The model under review builds one solid part; all positions refer to its coordinate system, in mm. A direction names the side the tool comes from. Round coordinates to 2 decimals unless told otherwise and drop trailing zeros. Write each loop counter-clockwise with the first axis right and the second up, starting at its lowest first coordinate (ties: lowest second). Pieces come first, ordered by that corner, then holes. Notation, with made-up numbers: M 4,54 L 10,54 A26 ccw 10,68 Z; hole C -18,38 d8. An arc over 180 degrees is marked long. Write item = value, one per line. Start each with the question number.
Item 1: Take a section at B-B, the plane y = 3.5. Give the boundary of the cut face in (x, z).
Item 2: Tool access review of faces 4 (the flat face through (0, 5, 0)), 5 (the flat face through (-1, 15, -14)), 6 (the cylindrical face through (17.553, 10.267, -2.764)): name each direction out of +Z, -Z, +X, -X, +Y, -Y from which nothing blocks a thin tool from reaching the whole face with its end or side.
Item 3: To check wall thickness, follow line 1 along X through (y, z) = (2.6, 0); line 2 along X through (y, z) = (7, 11.5); line 3 along X through (y, z) = (5.75, -7.5). State the ranges of each line that lie inside material, in increasing order.
Item 4: For pin 1 Ø5 at (x, z) = (38.5, -11.5) entering from -Y; pin 2 Ø3 at (x, z) = (61.5, 1) entering from -Y; pin 3 Ø13 at (x, z) = (60, 0) entering from +Y; pin 4 Ø7.5 at (x, z) = (-54.5, -1.5) entering from +Y, all flat-tipped, find the tip position at first contact; note any pin that passes through.
Item 5: Take a section at D-D, the plane x = 0. Give the boundary of the cut face in (y, z).
Item 6: Take a section at A-A, the plane x = -30. Give the boundary of the cut face in (y, z), plus the area to 3 significant figures.
Item 7: The part is to be moulded in two halves that separate along X. For faces 1 (the flat face through (75, 7, 0)), 2 (the flat face through (-1, 7, 15)), 3 (the cylindrical face through (-34.88, 2.46, -1.08)), say which applies: +X half, -X half, draft (parallel to the pull), parting line (faces both ways), or undercut.
Item 8: Take a section at C-C, the plane z = -9.25. Give the boundary of the cut face in (x, y), plus the area to 3 significant figures.
from build123d import *

# Parameters (mm, degrees)
SKETCH1_W           = 150
SKETCH1_H           = 30
SKETCH1_R           = 5
BOSS_EXTRUDE1_DEPTH = 5
SKETCH2_W           = 150
SKETCH2_H           = 30
BOSS_EXTRUDE2_DEPTH = 10
SKETCH3_R           = 12.75
CUT_EXTRUDE1_DEPTH  = 9
SKETCH3_3_R         = 12.75
CUT_EXTRUDE2_DEPTH  = 9.2
SKETCH3_4_R         = 12.75
CUT_EXTRUDE3_DEPTH  = 9.4
SKETCH3_5_R         = 12.75
CUT_EXTRUDE4_DEPTH  = 9.6
SKETCH3_6_R         = 12.75
CUT_EXTRUDE5_DEPTH  = 9.8


with BuildPart() as part:
    # Sketch1 → Boss-Extrude1 (new body)
    with BuildSketch(Plane(origin=(0, 0, 0), x_dir=(1, 0, 0), z_dir=(0, 1, 0))):
        Rectangle(SKETCH1_W, SKETCH1_H)
        with Locations(Location((-60, 0, 0), (0, 0, 270))):
            Circle(SKETCH1_R, mode=Mode.SUBTRACT)
        with Locations(Location((-30, 0, 0), (0, 0, 270))):
            Circle(SKETCH1_R, mode=Mode.SUBTRACT)
        with Locations(Location((0, 0, 0), (0, 0, 270))):
            Circle(SKETCH1_R, mode=Mode.SUBTRACT)
        with Locations(Location((30, 0, 0), (0, 0, 270))):
            Circle(SKETCH1_R, mode=Mode.SUBTRACT)
        with Locations(Location((60, 0, 0), (0, 0, 270))):
            Circle(SKETCH1_R, mode=Mode.SUBTRACT)
    extrude(amount=BOSS_EXTRUDE1_DEPTH)

    # Sketch2 → Boss-Extrude2 (add)
    with BuildSketch(Plane(origin=(0, 5, 0), x_dir=(1, 0, 0), z_dir=(0, 1, 0))):
        Rectangle(SKETCH2_W, SKETCH2_H)
    extrude(amount=BOSS_EXTRUDE2_DEPTH)

    # Sketch3 → Cut-Extrude1 (cut)
    with BuildSketch(Plane(origin=(0, 15, 0), x_dir=(1, 0, 0), z_dir=(0, 1, 0))):
        with Locations(Location((-60, 0, 0), (0, 0, 270))):
            Circle(SKETCH3_R)
    extrude(amount=-CUT_EXTRUDE1_DEPTH, mode=Mode.SUBTRACT)

    # Sketch3<3> → Cut-Extrude2 (cut)
    with BuildSketch(Plane(origin=(0, 15, 0), x_dir=(1, 0, 0), z_dir=(0, 1, 0))):
        with Locations(Location((-30, 0, 0), (0, 0, 270))):
            Circle(SKETCH3_3_R)
    extrude(amount=-CUT_EXTRUDE2_DEPTH, mode=Mode.SUBTRACT)

    # Sketch3<4> → Cut-Extrude3 (cut)
    with BuildSketch(Plane(origin=(0, 15, 0), x_dir=(1, 0, 0), z_dir=(0, 1, 0))):
        with Locations(Location((0, 0, 0), (0, 0, 270))):
            Circle(SKETCH3_4_R)
    extrude(amount=-CUT_EXTRUDE3_DEPTH, mode=Mode.SUBTRACT)

    # Sketch3<5> → Cut-Extrude4 (cut)
    with BuildSketch(Plane(origin=(0, 15, 0), x_dir=(1, 0, 0), z_dir=(0, 1, 0))):
        with Locations(Location((30, 0, 0), (0, 0, 270))):
            Circle(SKETCH3_5_R)
    extrude(amount=-CUT_EXTRUDE4_DEPTH, mode=Mode.SUBTRACT)

    # Sketch3<6> → Cut-Extrude5 (cut)
    with BuildSketch(Plane(origin=(0, 15, 0), x_dir=(1, 0, 0), z_dir=(0, 1, 0))):
        with Locations(Location((60, 0, 0), (0, 0, 270))):
            Circle(SKETCH3_6_R)
    extrude(amount=-CUT_EXTRUDE5_DEPTH, mode=Mode.SUBTRACT)


solid = part.part
Response values:
q1.outline = M -75,-15 L 75,-15 L 75,15 L -75,15 Z; hole C -60,0 d10; hole C -30,0 d10; hole C 0,0 d10; hole C 30,0 d10; hole C 60,0 d10
q2.face_4 = -Y
q2.face_5 = +Z, -Z, +X, -X, +Y
q2.face_6 = +Y
q3.line_1 = -75 to -65, -55 to -35, -25 to -5, 5 to 25, 35 to 55, 65 to 75
q3.line_2 = -75 to -65.51, -54.49 to -35.51, -24.49 to -5.51, 5.51 to 24.49, 35.51 to 54.49, 65.51 to 75
q3.line_3 = -75 to -10.31, 10.31 to 19.69, 40.31 to 49.69, 70.31 to 75
q4.pin_1 = 0
q4.pin_2 = 5
q4.pin_3 = 5.2
q4.pin_4 = 6
q5.outline = M 0,-15 L 15,-15 L 15,-12.75 L 5.6,-12.75 L 5.6,12.75 L 15,12.75 L 15,15 L 0,15 L 0,5 L 5,5 L 5,-5 L 0,-5 Z
q6.outline = M 0,-15 L 15,-15 L 15,-12.75 L 5.8,-12.75 L 5.8,12.75 L 15,12.75 L 15,15 L 0,15 L 0,5 L 5,5 L 5,-5 L 0,-5 Z
q6.area = 165 mm2
q7.face_1 = +X half
q7.face_2 = draft
q7.face_3 = undercut
q8.outline = M -75,0 L 75,0 L 75,15 L 68.77,15 L 68.77,5.2 L 51.23,5.2 L 51.23,15 L 38.77,15 L 38.77,5.4 L 21.23,5.4 L 21.23,15 L 8.77,15 L 8.77,5.6 L -8.77,5.6 L -8.77,15 L -21.23,15 L -21.23,5.8 L -38.77,5.8 L -38.77,15 L -51.23,15 L -51.23,6 L -68.77,6 L -68.77,15 L -75,15 Z
q8.area = 1,430 mm2
